Can you work these out from the model? Positions are in its coordinate system, mm. Face numbers are marked on the shaded views. A direction names the side the tool comes from. Coordinates: 2 decimals unless noted, no trailing zeros. Order: outer loops, then holes, each group sorted by start corner. A loop starts at its lowest first (then second) coordinate and runs counter-clockwise, first axis right, second up. Notation, with made-up numbers: M 12,-3 L 21,-3 A30 ccw 21,33 Z; hole C 26,-34 d3. An arc over 180 degrees is marked long. Answer as CSV lines item,"result". Start each with the question number.
1. If we section it at A-A (x = 24): List the corners of the cut face in (y, z) for me.
2. Will these pins go through, and if not, where does the flat tip stop? pin 1 (10 mm diameter, centred on x = 95, z = 103, fed in from +Y); pin 2 (10 mm diameter, centred on x = -66, z = 157.5, fed in from -Y); pin 3 (6 mm diameter, centred on x = 95, z = 82.5, fed in from +Y); pin 4 (12 mm diameter, centred on x = -73, y = -1.5, fed in from -Z).
3. If we section it at B-B (y = 74.5): List the corners of the cut face in (x, z) for me, plus the area to 3 significant figures.
4. If we section it at C-C (z = 64): List the corners of the cut face in (x, y) for me, plus the area to 3 significant figures.
5. I need wall thicknesses on line 1 along Z through (x, y) = (-138.5, 45); line 2 along Y through (x, z) = (72, 113.5); line 3 along Y through (x, z) = (-52, 63.5). Which ranges of each line are inside material? Lowest first, please. Write a range as from..to.
6. On a 3-axis mill with a long thin cutter (end or side, diameter ignored), from which of +Z, -Z, +X, -X, +Y, -Y can I reach the whole of each face in a straight line? I mean the marked faces 1 and 2. Say none if no direction works.
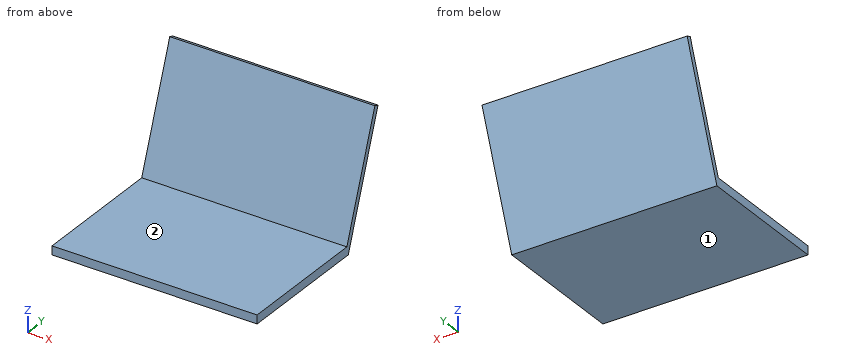
```python
from build123d import *

# Parameters (mm, degrees)
SKETCH_W     = 330
SKETCH_H     = 220
PAD_DEPTH    = 14
PAD001_DEPTH = 165


with BuildPart() as part:
    # Sketch → Pad (new body)
    with BuildSketch(Plane.XY):
        Rectangle(SKETCH_W, SKETCH_H)
    extrude(amount=PAD_DEPTH)

    # Sketch001 → Pad001 (join, symmetric)
    with BuildSketch(Plane.YZ):
        Polygon((110, 0), (181.824324, 197.335416), (174.306784, 200.071581), (102.48246, 2.736165), align=None)
    extrude(amount=PAD001_DEPTH, both=True)


solid = part.part
```
Solved:
1,outline,"M -110,0 L 110,0 L 181.82,197.34 L 174.31,200.07 L 106.58,14 L -110,14 Z"
2,pin 1,"y = 149.31"
2,pin 2,"y = 156.99"
2,pin 3,"y = 141.12"
2,pin 4,"z = 0"
3,outline,"M -165,0 L 165,0 L 165,14 L -165,14 Z"
3,area,"4,620 mm²"
4,outline,"M -165,124.78 L 165,124.78 L 165,133.29 L -165,133.29 Z"
4,area,"2,810 mm²"
5,line 1,"0..14"
5,line 2,"142.8..151.31"
5,line 3,"124.6..133.11"
6,face 1,"-Z, +X, -X, +Y, -Y"
6,face 2,"+Z, +X, -X, -Y"
